For this review, take the finished solid that the model builds, in its own axes (mm). Face numbers are marked on the shaded views. A direction names the side the tool comes from. Give positions to 0.01 mm unless a question says otherwise; leave off trailing zeros. Order: outer loops, then holes, each group sorted by start corner. A loop starts at its lowest first (then second) coordinate and runs counter-clockwise, first axis right, second up. Notation, with made-up numbers: M 46,19.5 L 57,19.5 A26 ccw 57,47.5 Z; hole C 18,19.25 d3. An arc over 180 degrees is marked long. Use CSV: the item, a comma, the result in double quotes. Start each with the question number.
(1) Draft analysis for pull direction Z (two halves, no side actions). For the marked faces 6, 7 and 8, state which applies: pulls with the +Z half, pulls with the -Z half, needs draft (parallel to the pull), parting line crosses it, or undercut.
(2) Consider section B-B (x = -25.5). Write out the cut boundary in (y, z), and give its area (3 significant figures).
(3) Consider section A-A (y = 11). Write out the cut boundary in (x, z).
(4) Wall thickness on L1, parallel to Y at x = 4.5, z = -3.5; L2, parallel to X at y = 6, z = -23; L3, parallel to X at y = 10.5, z = -27.5: over which ranges is each line inside the solid? List them lowest first. Write a range as from..to.
(5) Clearance check with flat-ended pins moving along their axes: P1, Ø2, axis at x = -19.5, y = 9, coming from the -Z side; P2, Ø3.5, axis at x = 25, y = 12.5, coming from the -Z side; P3, Ø8, axis at y = 10, z = -24, coming from the -X side. State where each tip first meets the part, or that it passes through.
(6) Tool access review of the marked faces 1, 2, 3, 4 and 5: name each direction out of +Z, -Z, +X, -X, +Y, -Y from which nothing blocks a thin tool from reaching the whole face with its end or side.
(7) Consider section C-C (z = -5). Write out the cut boundary in (x, y).
(8) Consider section D-D (x = -11.5). Write out the cut boundary in (y, z), and give its area (3 significant figures).
```python
from build123d import *

# Parameters (mm, degrees)
SKETCH1_W            = 76.2
SKETCH1_H            = 76.2
BOSS_EXTRUDE1_DEPTH  = 5.08
BOSS_EXTRUDE2_DEPTH  = 12.7
LPATTERN1_COUNT      = 2
LPATTERN1_PITCH      = 50.8
LPATTERN1_COUNT_DIR2 = 2
LPATTERN1_PITCH_DIR2 = 48.26


with BuildPart() as part:
    # Sketch1 → Boss-Extrude1 (new body)
    with BuildSketch(Plane(origin=(0, 0, 0), x_dir=(1, 0, 0), z_dir=(0, 1, 0))):
        Rectangle(SKETCH1_W, SKETCH1_H)
    extrude(amount=BOSS_EXTRUDE1_DEPTH)

    # Sketch2 → Boss-Extrude2 (add)
    with BuildSketch(Plane(origin=(0, 5.08, 0), x_dir=(1, 0, 0), z_dir=(0, 1, 0))):
        Polygon((-21.733825791, 19.05), (-18.067651581, 25.4), (-21.733825791, 31.75), (-29.066174209, 31.75), (-32.732348419, 25.4), (-29.066174209, 19.05), align=None)
    boss_extrude2 = extrude(amount=BOSS_EXTRUDE2_DEPTH)

    # LPattern1: Boss-Extrude2 2 × 2
    with Locations(*[(i * LPATTERN1_PITCH, 0, j * LPATTERN1_PITCH_DIR2) for i in range(LPATTERN1_COUNT) for j in range(LPATTERN1_COUNT_DIR2) if (i, j) != (0, 0)]):
        add(boss_extrude2)


solid = part.part
```
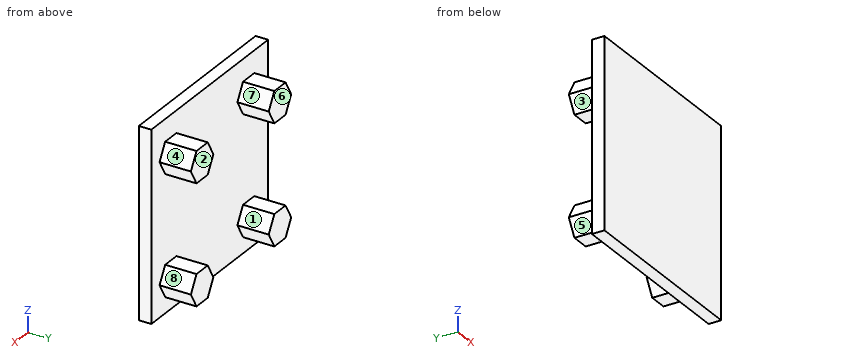
Check result:
1,face 6,"needs draft"
1,face 7,"pulls with the +Z half"
1,face 8,"undercut"
2,outline,"M 0,-38.1 L 5.08,-38.1 L 5.08,-31.75 L 17.78,-31.75 L 17.78,-19.05 L 5.08,-19.05 L 5.08,16.51 L 17.78,16.51 L 17.78,29.21 L 5.08,29.21 L 5.08,38.1 L 0,38.1 Z"
2,area,"710 mm^2"
3,outline,"M -32.73,-25.4 L -29.07,-31.75 L -21.73,-31.75 L -18.07,-25.4 L -21.73,-19.05 L -29.07,-19.05 Z; M -32.73,22.86 L -29.07,16.51 L -21.73,16.51 L -18.07,22.86 L -21.73,29.21 L -29.07,29.21 Z; M 18.07,-25.4 L 21.73,-31.75 L 29.07,-31.75 L 32.73,-25.4 L 29.07,-19.05 L 21.73,-19.05 Z; M 18.07,22.86 L 21.73,16.51 L 29.07,16.51 L 32.73,22.86 L 29.07,29.21 L 21.73,29.21 Z"
4,L1,"y = 0..5.08"
4,L2,"x = -31.35..-19.45, 19.45..31.35"
4,L3,"x = -31.52..-19.28, 19.28..31.52"
5,P1,"stops at z = -29.61"
5,P2,"stops at z = -31.75"
5,P3,"stops at x = -32.73"
6,face 1,"+Y"
6,face 2,"+Z, -Z, +X, -X, +Y"
6,face 3,"-X, +Y"
6,face 4,"+Z, +X, +Y"
6,face 5,"-Z, -X, +Y"
7,outline,"M -38.1,0 L 38.1,0 L 38.1,5.08 L -38.1,5.08 Z"
8,outline,"M 0,-38.1 L 5.08,-38.1 L 5.08,38.1 L 0,38.1 Z"
8,area,"387 mm^2"
